CAD build for the part. Positions are in the model's coordinates, mm. Face numbers are marked on the shaded views. Give positions to 0.01 mm unless a question says otherwise; leave off trailing zeros. Write each loop counter-clockwise with the first axis right and the second up, starting at its lowest first coordinate (ties: lowest second). Pieces come first, ordered by that corner, then holes. Notation, with made-up numbers: M 0,56.5 L 9,56.5 A29 cw 9,95.5 Z; hole C 81.5,27.5 d11. An arc over 180 degrees is marked long. One line per question, with ' | ' between items. Start each with the question number.
1. Pull direction X, two halves, no side cores. Call the marked faces 1, 2 and 3: released by +X, released by -X, zero draft, split by the parting line, or undercut.
2. Wall check: L1, parallel to X at y = 9, z = 0; L2, parallel to X at y = 5.75, z = -11. Give the ranges that are in metal, low to high.
3. Cut at C-C, the plane z = 0. Write the cut outline in (x, y).
4. Cut at D-D, the plane z = -11. Write the cut outline in (x, y).
5. Cut at A-A, the plane y = 4. Write the cut outline in (x, z), then the cut area to 3 significant figures.
6. Cut at B-B, the plane x = 0. Write the cut outline in (y, z).
7. Flat gauge pins, fed straight in: pin 1 (2.5 mm diameter, centred on x = 11, z = 10.5, fed in from -Y); pin 2 (1.5 mm diameter, centred on x = -11, z = -11, fed in from -Y); pin 3 (4 mm diameter, centred on y = 3, z = 19, fed in from +X). Where does each tip first touch, or does it go through?
```python
from build123d import *

# Parameters (mm, degrees)
SKETCH1_R           = 24
BOSS_EXTRUDE1_DEPTH = 13
SKETCH2_R           = 5
CUT_EXTRUDE1_DEPTH  = 10
SKETCH3_R           = 1.5
CUT_EXTRUDE2_DEPTH  = 8


with BuildPart() as part:
    # Sketch1 → Boss-Extrude1 (new body)
    with BuildSketch(Plane(origin=(0, 0, 0), x_dir=(1, 0, 0), z_dir=(0, 1, 0))):
        Circle(SKETCH1_R)
    extrude(amount=BOSS_EXTRUDE1_DEPTH)

    # Sketch2 → Cut-Extrude1 (cut)
    with BuildSketch(Plane(origin=(0, 13, 0), x_dir=(1, 0, 0), z_dir=(0, 1, 0))):
        Circle(SKETCH2_R)
    extrude(amount=-CUT_EXTRUDE1_DEPTH, mode=Mode.SUBTRACT)

    # Sketch3 → Cut-Extrude2 (cut)
    with BuildSketch(Plane(origin=(0, 0, 0), x_dir=(-1, 0, 0), z_dir=(0, -1, 0))):
        with BuildLine():
            ThreePointArc((11, -9.5), (9.939339828, -9.939339828), (9.5, -11))
            Line((9.5, -11), (11, -11))
            Line((11, -11), (11, -9.5))
        make_face()
        with BuildLine():
            Line((11, -11), (9.5, -11))
            ThreePointArc((9.5, -11), (11, -12.5), (12.5, -11))
            ThreePointArc((12.5, -11), (12.060660172, -9.939339828), (11, -9.5))
            Line((11, -9.5), (11, -11))
        make_face()
        with BuildLine():
            ThreePointArc((-11, -9.5), (-12.060660172, -12.060660172), (-9.5, -11))
            Line((-9.5, -11), (-11, -11))
            Line((-11, -11), (-11, -9.5))
        make_face()
        with BuildLine():
            Line((-11, -11), (-9.5, -11))
            ThreePointArc((-9.5, -11), (-9.939339828, -9.939339828), (-11, -9.5))
            Line((-11, -9.5), (-11, -11))
        make_face()
        with Locations((11, 11)):
            Circle(SKETCH3_R)
        with Locations((-11, 11)):
            Circle(SKETCH3_R)
    extrude(amount=-CUT_EXTRUDE2_DEPTH, mode=Mode.SUBTRACT)


solid = part.part
```
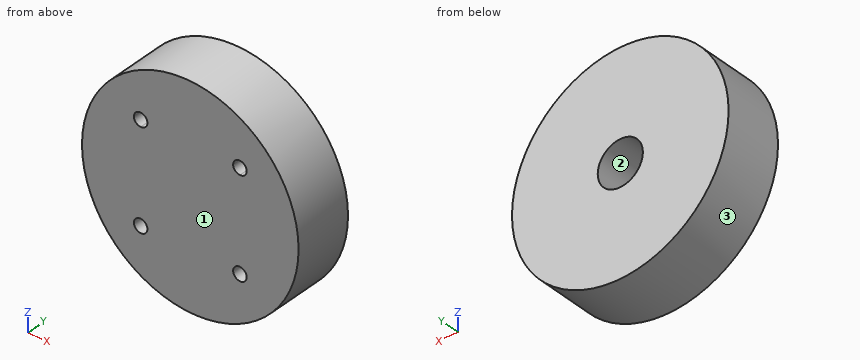
Here are the results:
1) face 1: zero draft | face 2: undercut | face 3: split by the parting line
2) L1: -24 to -5, 5 to 24 | L2: -21.33 to -12.5, -9.5 to 9.5, 12.5 to 21.33
3) outline: M -24,0 L 24,0 L 24,13 L 5,13 L 5,3 L -5,3 L -5,13 L -24,13 Z
4) outline: M -21.33,0 L -12.5,0 L -12.5,8 L -9.5,8 L -9.5,0 L 9.5,0 L 9.5,8 L 12.5,8 L 12.5,0 L 21.33,0 L 21.33,13 L -21.33,13 Z
5) outline: C 0,0 d48; hole C -11,-11 d3; hole C -11,11 d3; hole C 0,0 d10; hole C 11,-11 d3; hole C 11,11 d3 | area: 1,700 mm^2
6) outline: M 0,-24 L 13,-24 L 13,-5 L 3,-5 L 3,5 L 13,5 L 13,24 L 0,24 Z
7) pin 1: y = 0 | pin 2: y = 8 | pin 3: x = 16.94
